from build123d import *

# Parameters (mm, degrees)
F0_W     = 15
F0_H     = 12.9903810568
F1_DEPTH = 40
F4_T     = -2.5
F5_DEPTH = 25
F6_DEPTH = 25
F7_R     = 4.25
F8_DEPTH = 40


with BuildPart() as f1:
    # F0 (on Front) → F1 (new body)
    with BuildSketch(Plane.XZ):
        Polygon((30, 25), (15, 25), (0, -0.9807621135), (-15, 25), (-30, 25), (-30, -25), (30, -25), align=None)
        Polygon((7.5, 37.9903810568), (7.5, 25), (15, 25), (18.75, 31.4951905284), align=None)
        with Locations((0, 31.4951905284)):
            Rectangle(F0_W, F0_H)
        Polygon((-15, 25), (-7.5, 25), (-7.5, 37.9903810568), (-18.75, 31.4951905284), align=None)
        Polygon((-30, 25), (-15, 25), (-18.75, 31.4951905284), align=None)
        Polygon((18.75, 31.4951905284), (15, 25), (30, 25), align=None)
        Polygon((15, 25), (7.5, 25), (-7.5, 25), (-15, 25), (0, -0.9807621135), align=None)
    extrude(amount=F1_DEPTH)

    # F4
    f4_openings = [f1.faces().sort_by_distance(p)[0] for p in [
        (0, -20, -25),
    ]]
    offset(amount=F4_T, openings=f4_openings)

    # F3 (on face) → F5 (cut)
    with BuildSketch(Plane(origin=(18.3253175473, 0, 31.7403810568), x_dir=(0.8660254038, 0, -0.5), z_dir=(0.5, 0, 0.8660254038))):
        with BuildLine():
            ThreePointArc((9.4903810568, -24.1), (-5.8735799739, -17.7360389693), (0.4903810568, -33.1))
            ThreePointArc((0.4903810568, -33.1), (6.8543420874, -30.4639610307), (9.4903810568, -24.1))
        make_face()
    extrude(amount=-F5_DEPTH, mode=Mode.SUBTRACT)

    # F2 (on face) → F6 (cut)
    with BuildSketch(Plane(origin=(-18.3253175473, 0, 31.7403810568), x_dir=(0.8660254038, 0, 0.5), z_dir=(-0.5, 0, 0.8660254038))):
        with BuildLine():
            ThreePointArc((8.5096189432, -15.9), (5.8735799739, -9.5360389693), (-0.4903810568, -6.9))
            ThreePointArc((-0.4903810568, -6.9), (-6.8543420874, -22.2639610307), (8.5096189432, -15.9))
        make_face()
    extrude(amount=-F6_DEPTH, mode=Mode.SUBTRACT)

    # F7 (on face) → F8 (cut)
    with BuildSketch(Plane.XZ.offset(40)):
        with Locations((0, -0.9807621135)):
            Circle(F7_R)
    extrude(amount=-F8_DEPTH, mode=Mode.SUBTRACT)


solid = f1.part
Work out the finished part from the listing and answer in its coordinate system (mm). A direction names the side the tool comes from. Round coordinates to 2 decimals unless told otherwise and drop trailing zeros. Write each loop counter-clockwise with the first axis right and the second up, starting at its lowest first coordinate (ties: lowest second). Pieces come first, ordered by that corner, then holes. Notation, with made-up numbers: (0.25, -34.5) -> (32.25, -34.5) arc R21 ccw to (32.25, -4.5) -> close; hole circle Ø3 at (-20.75, 35.25). An arc over 180 degrees is marked (long way). Write each question's results on one line, items separated by ' | '.
Item 1: A cutting plane is placed at B-B, the plane y = -9. Determine the outline of the cut face in (x, z).
Result set:
outline: (-30, -25) -> (-27.5, -25) -> (-27.5, 23.56) -> (-22.5, 26.44) -> (-23.75, 28.61) -> (-30, 25) -> close; (-13.75, 34.38) -> (-12.5, 32.22) -> (-6.83, 35.49) -> (6.83, 35.49) -> (27.5, 23.56) -> (27.5, -25) -> (30, -25) -> (30, 25) -> (7.5, 37.99) -> (-7.5, 37.99) -> close
Item 2: The mould has two halves that part along X. Classify faces 1 (the face through (21.41, -15.28, 29.96)), 2 (the face through (-27.5, -20, 0)), 3 (the face through (-0.92, -38.77, -5.13)), 4 (the face through (-30, -20, 0)): +X half, -X half, draft (parallel to the pull), parting line (faces both ways), or undercut.
Result set:
face 1: +X half | face 2: undercut | face 3: undercut | face 4: -X half
Item 3: A cutting plane is placed at A-A, the plane x = 0. Determine the outline of the cut face in (y, z).
Result set:
outline: (-40, -25) -> (-37.5, -25) -> (-37.5, -5.23) -> (-40, -5.23) -> close; (-40, 3.27) -> (-37.5, 3.27) -> (-37.5, 35.49) -> (-2.5, 35.49) -> (-2.5, 3.27) -> (0, 3.27) -> (0, 37.99) -> (-40, 37.99) -> close; (-2.5, -25) -> (0, -25) -> (0, -5.23) -> (-2.5, -5.23) -> close
Item 4: A cutting plane is placed at D-D, the plane x = -6. Determine the outline of the cut face in (y, z), plus the area to 3 significant figures.
Result set:
outline: (-40, -25) -> (-37.5, -25) -> (-37.5, 35.49) -> (-2.5, 35.49) -> (-2.5, -25) -> (0, -25) -> (0, 37.99) -> (-40, 37.99) -> close | area: 402 mm^2
Item 5: Which of the six approach directions +Z, -Z, +X, -X, +Y, -Y give full straight-line access (tool end or side, diameter ignored) to faces 5 (the face through (0, -37.5, 6)), 6 (the face through (0, -20, 37.99))?
Result set:
face 5: -Z | face 6: +Z, +X, -X, +Y, -Y
Item 6: A cutting plane is placed at C-C, the plane z = -2.5. Determine the outline of the cut face in (x, y).
Result set:
outline: (-30, -40) -> (-3.97, -40) -> (-3.97, -37.5) -> (-27.5, -37.5) -> (-27.5, -2.5) -> (-3.97, -2.5) -> (-3.97, 0) -> (-30, 0) -> close; (3.97, -40) -> (30, -40) -> (30, 0) -> (3.97, 0) -> (3.97, -2.5) -> (27.5, -2.5) -> (27.5, -37.5) -> (3.97, -37.5) -> close
Item 7: Find the intervals of material crossed by line 1 along Y through (x, z) = (-22, -10); line 2 along X through (y, z) = (-24.5, -21); line 3 along Z through (x, y) = (0, -39), in increasing order. Write a range as [from, to].
Result set:
line 1: [-40, -37.5], [-2.5, 0] | line 2: [-30, -27.5], [27.5, 30] | line 3: [-25, -5.23], [3.27, 37.99]
Item 8: Flat-ended cylindrical pins translate along their axes: P1, Ø1.5, axis at x = 9, y = -16, coming from the +Z side; P2, Ø2, axis at x = 23, y = -8, coming from the +Z side; P3, Ø12, axis at x = 2, y = -19, coming from the -Z side; P4, Ø7, axis at x = 0, z = -0.98, coming from the +Y side. Find the tip coordinate at first contact, or state that the pin passes through.
Result set:
P1: z = 37.56 | P2: z = 29.62 | P3: z = 34.81 | P4: through
